Check sheet for the modelled part. Datum: model origin and axes. Units: mm. A direction names the side the tool comes from. Round coordinates to 2 decimals unless told otherwise and drop trailing zeros. Write each loop counter-clockwise with the first axis right and the second up, starting at its lowest first coordinate (ties: lowest second). Pieces come first, ordered by that corner, then holes. Notation, with made-up numbers: (-25, 0.5) -> (-1, 0.5) arc R16 ccw to (-1, 15.5) -> close; hole circle Ø6 at (4, -9). An arc over 180 degrees is marked (long way). Write item = value, one per line.
from build123d import *

# Parameters (mm, degrees)
EXTRUSION1_DEPTH = 40
ESQUISSE2_R      = 1.5
EXTRUSION2_DEPTH = 10
ESQUISSE6_R      = 1.5
EXTRUSION6_DEPTH = 10


with BuildPart() as part:
    # Esquisse1 → Extrusion1 (new body)
    with BuildSketch(Plane.XY):
        Polygon((-17.090791643, 12.954), (-17.090791643, -2.046), (2.909208357, -2.046), (2.909208357, 12.954), (1.409208357, 12.954), (1.409208357, -0.546), (-15.590791643, -0.546), (-15.590791643, 12.954), align=None)
    extrude(amount=EXTRUSION1_DEPTH)

    # Esquisse2 → Extrusion2 (cut)
    with BuildSketch(Plane(origin=(2.909208357, 0, 0), x_dir=(0, 0, -1), z_dir=(1, 0, 0))):
        with Locations((-18, 5.454)):
            Circle(ESQUISSE2_R)
        with Locations((-4, 5.454)):
            Circle(ESQUISSE2_R)
        Polygon((-40, 12.954), (-28, 12.954), (-40, 7.954), align=None)
    extrude(amount=-EXTRUSION2_DEPTH, mode=Mode.SUBTRACT)

    # Esquisse6 → Extrusion6 (cut)
    with BuildSketch(Plane.ZY.offset(17.090791643)):
        with Locations(Location((31, 7.954, 0), (0, 0, 270))):
            Circle(ESQUISSE6_R)
        with Locations(Location((16, 7.954, 0), (0, 0, 270))):
            Circle(ESQUISSE6_R)
    extrude(amount=-EXTRUSION6_DEPTH, mode=Mode.SUBTRACT)


solid = part.part
(1) Sectioned sample at C-C on y = 11.75. Enter the section's corners in (x, z), then the cut area to 3 significant figures.
Worked answers:
outline = (-17.09, 0) -> (-15.59, 0) -> (-15.59, 40) -> (-17.09, 40) -> close; (1.41, 0) -> (2.91, 0) -> (2.91, 30.89) -> (1.41, 30.89) -> close
area = 106 mm²
(2) Sectioned sample at A-A on z = 18. Enter the section's corners in (x, y), then the cut area to 3 significant figures.
Worked answers:
outline = (-17.09, -2.05) -> (2.91, -2.05) -> (2.91, 3.95) -> (1.41, 3.95) -> (1.41, -0.55) -> (-15.59, -0.55) -> (-15.59, 12.95) -> (-17.09, 12.95) -> close; (1.41, 6.95) -> (2.91, 6.95) -> (2.91, 12.95) -> (1.41, 12.95) -> close
area = 66.0 mm²
(3) Material ranges on L1, parallel to X at y = 8, z = 9; L2, parallel to Y at x = 1.8, z = 4; L3, parallel to X at y = 12.5, z = 31, recorded low to high. Write a range as [from, to].
Worked answers:
L1 = [-17.09, -15.59], [1.41, 2.91]
L2 = [-2.05, 3.95], [6.95, 12.95]
L3 = [-17.09, -15.59]
(4) Access from +Z, -Z, +X, -X, +Y, -Y to the whole of each face (thin tool, end or side, straight path). Record for faces 1 (the flat face through (-6, -1, 0)), 2 (the cylindrical face through (-16.351, 9.453, 31.066)), 3 (the cylindrical face through (2.2, 5.5, 19.5)), 4 (the flat face through (-7, -0.546, 20)), 5 (the flat face through (-9, -1, 40)).
Worked answers:
face_1 = -Z, +X, -X, +Y, -Y
face_2 = -X
face_3 = +X
face_4 = +Z, -Z, +Y
face_5 = +Z, +X, -X, +Y, -Y
(5) Sectioned sample at B-B on z = 10. Enter the section's corners in (x, y), then the cut area to 3 significant figures.
Worked answers:
outline = (-17.09, -2.05) -> (2.91, -2.05) -> (2.91, 12.95) -> (1.41, 12.95) -> (1.41, -0.55) -> (-15.59, -0.55) -> (-15.59, 12.95) -> (-17.09, 12.95) -> close
area = 70.5 mm²
(6) Release check for a two-part mould opening along Y. For faces 6 (the flat face through (2.17, 10.489, 33.916)), 7 (the cylindrical face through (-16.351, 9.453, 16.066)), 8 (the flat face through (-7, -2.046, 20)) record: pulls with the +Y half, pulls with the -Y half, needs draft (parallel to the pull), parting line crosses it, or undercut.
Worked answers:
face_6 = pulls with the +Y half
face_7 = undercut
face_8 = pulls with the -Y half
(7) Go/stop test with a flat-tipped pin: P1, Ø6, axis at x = -8, z = 32.5, coming from the +Y side. Record where the tip stops, or that it passes through.
Worked answers:
P1 = -0.55
(8) Sectioned sample at D-D on x = -11.5. Enter the section's corners in (y, z).
Worked answers:
outline = (-2.05, 0) -> (-0.55, 0) -> (-0.55, 40) -> (-2.05, 40) -> close
